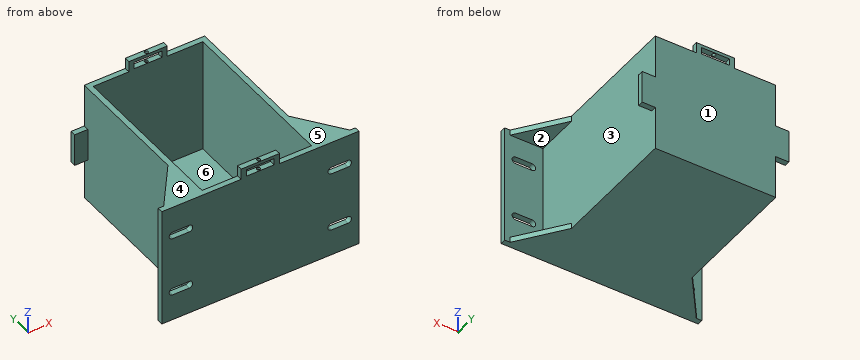
from build123d import *

# Parameters (mm, degrees)
SKETCH1_W           = 110
SKETCH1_H           = 162
BOSS_EXTRUDE1_DEPTH = 55
SHELL1_T            = -5
SKETCH2_W           = 35
SKETCH2_H           = 5
BOSS_EXTRUDE2_DEPTH = 55
BOSS_EXTRUDE3_DEPTH = 55
SKETCH12_W          = 35
SKETCH12_H          = 40
CUT_EXTRUDE5_DEPTH  = 50
CUT_EXTRUDE1_DEPTH  = 5
SKETCH6_W           = 12
SKETCH6_H           = 5
BOSS_EXTRUDE4_DEPTH = 15
SKETCH7_W           = 10
SKETCH7_H           = 5
BOSS_EXTRUDE5_DEPTH = 17.5
CUT_EXTRUDE2_START  = -162
SKETCH8_W           = 25.3
SKETCH8_H           = 6.2
CUT_EXTRUDE2_DEPTH  = 162
SKETCH9_R           = 1.6
CUT_EXTRUDE3_DEPTH  = 11


with BuildPart() as part:
    # Sketch1 → Boss-Extrude1 (new, symmetric)
    with BuildSketch(Plane.XY):
        Rectangle(SKETCH1_W, SKETCH1_H)
    extrude(amount=BOSS_EXTRUDE1_DEPTH, both=True)

    # Shell1
    shell1_openings = [part.faces().sort_by_distance(p)[0] for p in [
        (0, 0, 55),
    ]]
    offset(amount=SHELL1_T, openings=shell1_openings, kind=Kind.INTERSECTION)

    # Sketch2 → Boss-Extrude2 (add, symmetric)
    with BuildSketch(Plane.XY):
        with Locations((-72.5, -78.5)):
            Rectangle(SKETCH2_W, SKETCH2_H)
        with Locations((72.5, -78.5)):
            Rectangle(SKETCH2_W, SKETCH2_H)
    extrude(amount=BOSS_EXTRUDE2_DEPTH, both=True)

    # Sketch3 → Boss-Extrude3 (add, symmetric)
    with BuildSketch(Plane.XY):
        Polygon((-85, -76), (-55, -36), (-55, -76), align=None)
        Polygon((55, -36), (55, -76), (85, -76), align=None)
    extrude(amount=BOSS_EXTRUDE3_DEPTH, both=True)

    # Sketch12 → Cut-Extrude5 (cut, symmetric)
    with BuildSketch(Plane.XY):
        with Locations((-72.5, -56)):
            Rectangle(SKETCH12_W, SKETCH12_H)
        with Locations((72.5, -56)):
            Rectangle(SKETCH12_W, SKETCH12_H)
    extrude(amount=CUT_EXTRUDE5_DEPTH, both=True, mode=Mode.SUBTRACT)

    # Sketch5 → Cut-Extrude1 (cut)
    with BuildSketch(Plane(origin=(0, -76, 0), x_dir=(1, 0, 0), z_dir=(0, 1, 0))):
        with BuildLine():
            Line((-80, 30.75), (-65, 30.75))
            ThreePointArc((-65, 30.75), (-61.75, 27.5), (-65, 24.25))
            Line((-65, 24.25), (-80, 24.25))
            ThreePointArc((-80, 24.25), (-83.25, 27.5), (-80, 30.75))
        make_face()
        with BuildLine():
            Line((80, 30.75), (65, 30.75))
            ThreePointArc((65, 30.75), (61.75, 27.5), (65, 24.25))
            Line((65, 24.25), (80, 24.25))
            ThreePointArc((80, 24.25), (83.25, 27.5), (80, 30.75))
        make_face()
        with BuildLine():
            Line((80, -30.75), (65, -30.75))
            ThreePointArc((65, -30.75), (61.75, -27.5), (65, -24.25))
            Line((65, -24.25), (80, -24.25))
            ThreePointArc((80, -24.25), (83.25, -27.5), (80, -30.75))
        make_face()
        with BuildLine():
            Line((-80, -30.75), (-65, -30.75))
            ThreePointArc((-65, -30.75), (-61.75, -27.5), (-65, -24.25))
            Line((-65, -24.25), (-80, -24.25))
            ThreePointArc((-80, -24.25), (-83.25, -27.5), (-80, -30.75))
        make_face()
    extrude(amount=-CUT_EXTRUDE1_DEPTH, mode=Mode.SUBTRACT)

    # Sketch6 → Boss-Extrude4 (add, symmetric)
    with BuildSketch(Plane.XY):
        with Locations((-61, 78.5)):
            Rectangle(SKETCH6_W, SKETCH6_H)
        with Locations((61, 78.5)):
            Rectangle(SKETCH6_W, SKETCH6_H)
    extrude(amount=BOSS_EXTRUDE4_DEPTH, both=True)

    # Sketch7 → Boss-Extrude5 (add, symmetric)
    with BuildSketch(Plane(origin=(0, 0, 0), x_dir=(0, 0, -1), z_dir=(1, 0, 0))):
        with Locations((-60, 78.5)):
            Rectangle(SKETCH7_W, SKETCH7_H)
        with Locations((-60, -78.5)):
            Rectangle(SKETCH7_W, SKETCH7_H)
    extrude(amount=BOSS_EXTRUDE5_DEPTH, both=True)

    # Sketch8 → Cut-Extrude2 (cut)
    with BuildSketch(Plane(origin=(0, 81, 0), x_dir=(1, 0, 0), z_dir=(0, 1, 0)).offset(CUT_EXTRUDE2_START)):
        with Locations((0, -59.1)):
            Rectangle(SKETCH8_W, SKETCH8_H)
    extrude(amount=CUT_EXTRUDE2_DEPTH, mode=Mode.SUBTRACT)

    # Sketch9 → Cut-Extrude3 (cut)
    with BuildSketch(Plane.XY.offset(65)):
        with Locations((0, -78.5)):
            Circle(SKETCH9_R)
        with Locations(Location((0, 78.5, 0), (0, 0, 180))):
            Circle(SKETCH9_R)
    extrude(amount=-CUT_EXTRUDE3_DEPTH, mode=Mode.SUBTRACT)


solid = part.part
Here's how the part is built. I have some questions about the finished solid (model axes, mm). Face numbers are marked on the shaded views. A direction names the side the tool comes from. Round coordinates to 2 decimals unless told otherwise and drop trailing zeros. Order: outer loops, then holes, each group sorted by start corner. A loop starts at its lowest first (then second) coordinate and runs counter-clockwise, first axis right, second up. Notation, with made-up numbers: M 75,-32.5 L 119,-32.5 A22 cw 119,-20.5 Z; hole C 4.5,40 d5. An arc over 180 degrees is marked long. Return JSON: item names as keys, results as strings. Group by question number.
1. Please list where these lines run through material, in increasing order: probe 1 along Y at (x, z) = (0, 55.1); probe 2 along X at (y, z) = (-33.5, 45.5); probe 3 along Y at (x, z) = (-15.5, -6).
2. I'm going to push flat-ended pins straight in: pin 1 Ø2.5 at (y, z) = (-78.5, 58.5) entering from -X; pin 2 Ø2 at (y, z) = (-55.5, 9.5) entering from -X; pin 3 Ø6 at (y, z) = (-48.5, 23.5) entering from +X; pin 4 Ø1 at (x, y) = (56.5, -30) entering from -Z. Where does each tip first touch, or does it pass through?
3. If we section it at D-D on y = -51: List the corners of the cut face in (x, z) for me.
4. On a 3-axis mill with a long thin cutter (end or side, diameter ignored), from which of +Z, -Z, +X, -X, +Y, -Y can I reach the whole of each face in a straight line? I mean the marked faces 4, 5 and 6. Say none if no direction works.
5. If we section it at C-C on x = -71.5: List the corners of the cut face in (y, z) for me.
6. If we section it at A-A on z = 27.5: List the corners of the cut face in (x, y) for me.
7. If we mould it in two halves opening along Y, with no side actions, what happens to the marked faces 1, 2 and 3? For each: pulls with the +Y half, pulls with the -Y half, needs draft (parallel to the pull), parting line crosses it, or undercut.
8. If we section it at B-B on z = -34: List the corners of the cut face in (x, y) for me.
Reply:
{
 "1": {"probe 1": "-81 to -80.1, -76.9 to -76, 76 to 76.9, 80.1 to 81", "probe 2": "-55 to -50, 50 to 55", "probe 3": "-81 to -76, 76 to 81"},
 "2": {"pin 1": "x = -17.5", "pin 2": "x = -55", "pin 3": "x = 55", "pin 4": "through"},
 "3": {"outline": "M -66.25,-55 L 66.25,-55 L 66.25,-50 L 55,-50 L 55,50 L 66.25,50 L 66.25,55 L 50,55 L 50,-50 L -50,-50 L -50,55 L -66.25,55 L -66.25,50 L -55,50 L -55,-50 L -66.25,-50 Z"},
 "4": {"face 4": "+Z, -X, +Y, -Y", "face 5": "+Z, +X, +Y, -Y", "face 6": "+Z"},
 "5": {"outline": "M -81,-55 L -58,-55 L -58,-50 L -76,-50 L -76,-30.75 L -81,-30.75 Z; M -81,-24.25 L -76,-24.25 L -76,24.25 L -81,24.25 Z; M -81,30.75 L -76,30.75 L -76,50 L -58,50 L -58,55 L -81,55 Z"},
 "6": {"outline": "M -90,-81 L -83.25,-81 L -83.25,-76 L -90,-76 Z; M -61.75,-81 L 61.75,-81 L 61.75,-76 L 55,-76 L 55,81 L -55,81 L -55,-76 L -61.75,-76 Z; M 83.25,-81 L 90,-81 L 90,-76 L 83.25,-76 Z; hole M -50,-76 L 50,-76 L 50,76 L -50,76 Z"},
 "7": {"face 1": "pulls with the +Y half", "face 2": "needs draft", "face 3": "undercut"},
 "8": {"outline": "M -90,-81 L 90,-81 L 90,-76 L 55,-76 L 55,81 L -55,81 L -55,-76 L -90,-76 Z; hole M -50,-76 L 50,-76 L 50,76 L -50,76 Z"}
}
